Work out the finished part from the listing and answer in its coordinate system (mm). A direction names the side the tool comes from. Coordinates: 2 decimals unless noted, no trailing zeros. Order: outer loops, then holes, each group sorted by start corner. A loop starts at its lowest first (then second) coordinate and runs counter-clockwise, first axis right, second up. Notation, with made-up numbers: M -11.5,-29.5 L 2.5,-29.5 A23 cw 2.5,3.5 Z; hole C 42.5,24.5 d11. An arc over 180 degrees is marked long. Use a Markdown table: item, result.
from build123d import *

# Parameters (mm, degrees)
F0_W     = 15.24
F0_H     = 45.72
F0_W_2   = 40.64
F0_H_2   = 15.24
F1_DEPTH = 15.24
F2_DEPTH = 63.5
F3_DEPTH = 43.18
F4_R     = 10.16
F5_DEPTH = 15.24
F6_R     = 7.62
F7_DEPTH = 15.24


with BuildPart() as f1:
    # F0 (on Top) → F1 (new body)
    with BuildSketch(Plane.XY):
        with BuildLine():
            Line((15.24, 45.72), (15.24, 0))
            Line((15.24, 0), (86.36, 0))
            ThreePointArc((86.36, 0), (93.544205, -2.975795), (96.52, -10.16))
            Line((96.52, -10.16), (96.52, -22.86))
            Line((96.52, -22.86), (137.16, -22.86))
            Line((137.16, -22.86), (137.16, -5.08))
            ThreePointArc((137.16, -5.08), (122.281024, 30.841024), (86.36, 45.72))
            Line((86.36, 45.72), (15.24, 45.72))
        make_face()
        with BuildLine():
            ThreePointArc((48.26, 15.24), (40.64, 22.86), (48.26, 30.48))
            Line((48.26, 30.48), (71.12, 30.48))
            ThreePointArc((71.12, 30.48), (78.74, 22.86), (71.12, 15.24))
            Line((71.12, 15.24), (48.26, 15.24))
        make_face(mode=Mode.SUBTRACT)
        with Locations((7.62, 22.86)):
            Rectangle(F0_W, F0_H)
        with Locations((116.84, -30.48)):
            Rectangle(F0_W_2, F0_H_2)
    extrude(amount=F1_DEPTH)

    # F0 (on Top) → F2 (join)
    with BuildSketch(Plane.XY):
        with Locations((7.62, 22.86)):
            Rectangle(F0_W, F0_H)
    extrude(amount=F2_DEPTH)

    # F0 (on Top) → F3 (join)
    with BuildSketch(Plane.XY):
        with Locations((116.84, -30.48)):
            Rectangle(F0_W_2, F0_H_2)
    extrude(amount=-F3_DEPTH)

    # F4 (on face) → F5 (cut, through all)
    with BuildSketch(Plane(origin=(0, 0, 0), x_dir=(0, -1, 0), z_dir=(-1, 0, 0))):
        with BuildLine():
            ThreePointArc((-22.86, 63.5), (-6.695539, 56.804461), (0, 40.64))
            Line((0, 40.64), (0, 63.5))
            Line((0, 63.5), (-22.86, 63.5))
        make_face()
        with BuildLine():
            Line((-45.72, 63.5), (-45.72, 40.64))
            ThreePointArc((-45.72, 40.64), (-39.024461, 56.804461), (-22.86, 63.5))
            Line((-22.86, 63.5), (-45.72, 63.5))
        make_face()
        with Locations((-22.86, 40.64)):
            Circle(F4_R)
    extrude(amount=-F5_DEPTH, mode=Mode.SUBTRACT)

    # F6 (on face) → F7 (cut, through all)
    with BuildSketch(Plane.XZ.offset(38.1)):
        with BuildLine():
            ThreePointArc((137.16, -22.86), (131.20841, -37.22841), (116.84, -43.18))
            Line((116.84, -43.18), (137.16, -43.18))
            Line((137.16, -43.18), (137.16, -22.86))
        make_face()
        with BuildLine():
            ThreePointArc((116.84, -43.18), (102.47159, -37.22841), (96.52, -22.86))
            Line((96.52, -22.86), (96.52, -43.18))
            Line((96.52, -43.18), (116.84, -43.18))
        make_face()
        with Locations((116.84, -22.86)):
            Circle(F6_R)
    extrude(amount=-F7_DEPTH, mode=Mode.SUBTRACT)


solid = f1.part
1. For a pull along X with two mould halves and no side action, classify faces 6 (the face through (78.74, 23.03, 7.51)), 7 (the face through (7.51, 25.06, 30.72)), 8 (the face through (122.674, 30.444, 7.513)) as +X half, -X half, draft (parallel to the pull), parting line (faces both ways), or undercut.
Answers below:
| item | result |
|---|---|
| face 6 | undercut |
| face 7 | draft |
| face 8 | +X half |
2. Flat-ended cylindrical pins translate along their axes: P1, Ø10, axis at y = 37, z = 0.5, coming from the +X side; P2, Ø23.5, axis at y = 22.86, z = 40.64, coming from the -X side; P3, Ø5, axis at x = 36, z = 14, coming from the -Y side; P4, Ø12, axis at x = 119.5, z = -27.5, coming from the +Y side. Find the tip coordinate at first contact, or state that the pin passes through.
Answers below:
| item | result |
|---|---|
| P1 | x = 121.08 |
| P2 | x = 0 |
| P3 | y = 0 |
| P4 | y = -22.86 |
3. Section A-A on y = -32 is taken. Determine the outline of the cut face in (x, z), then the cut area to 3 significant figures.
Answers below:
| item | result |
|---|---|
| outline | M 96.52,-22.86 A20.32 ccw 116.84,-43.18 A20.32 ccw 137.16,-22.86 L 137.16,15.24 L 96.52,15.24 Z; hole C 116.84,-22.86 d15.24 |
| area | 2,010 mm² |
4. Section C-C on z = -6.5 is taken. Determine the outline of the cut face in (x, y), then the cut area to 3 significant figures.
Answers below:
| item | result |
|---|---|
| outline | M 96.52,-38.1 L 137.16,-38.1 L 137.16,-22.86 L 96.52,-22.86 Z |
| area | 619 mm² |
5. Find the intervals of material crossed by probe 1 along Z at (x, y) = (5, 22); probe 2 along Z at (x, y) = (116.84, -29); probe 3 along Y at (x, z) = (7, 21), in increasing order.
Answers below:
| item | result |
|---|---|
| probe 1 | 0 to 30.52, 50.76 to 63.48 |
| probe 2 | -43.18 to -30.48, -15.24 to 15.24 |
| probe 3 | 0 to 45.72 |
6. Section D-D on x = 32.5 is taken. Determine the outline of the cut face in (y, z), then the cut area to 3 significant figures.
Answers below:
| item | result |
|---|---|
| outline | M 0,0 L 45.72,0 L 45.72,15.24 L 0,15.24 Z |
| area | 697 mm² |
7. Section B-B on x = 46.5 is taken. Determine the outline of the cut face in (y, z).
Answers below:
| item | result |
|---|---|
| outline | M 0,0 L 15.45,0 L 15.45,15.24 L 0,15.24 Z; M 30.27,0 L 45.72,0 L 45.72,15.24 L 30.27,15.24 Z |
8. For faces 1 (the face through (60, 30.48, 8)), 2 (the face through (117, -38.1, -14)), 3 (the face through (96.52, -27, 1)), 4 (the face through (121, -22.86, -16)), 5 (the face through (15.24, 23, 28)), determine the directions among +Z, -Z, +X, -X, +Y, -Y from which every point of the face is accessible in a straight line to the end or side of a thin tool.
Answers below:
| item | result |
|---|---|
| face 1 | +Z, -Z |
| face 2 | +Z, -Z, +X, -X, -Y |
| face 3 | +Z, -Z, -X, -Y |
| face 4 | -Z, +X, -X, +Y |
| face 5 | +Z, +X, +Y, -Y |
